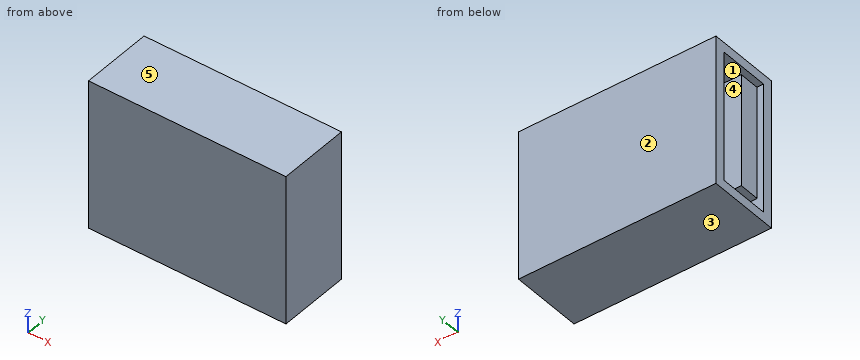
```python
from build123d import *

# Parameters (mm, degrees)
F0_W     = 19.3
F0_H     = 14.6
F1_DEPTH = 7
F2_W     = 5
F2_H     = 12.7
F3_DEPTH = 10
F4_W     = 2
F4_H     = 11
F5_DEPTH = 10


with BuildPart() as f1:
    # F0 (on Front) → F1 (new body)
    with BuildSketch(Plane.XZ):
        with Locations((9.65, 7.3)):
            Rectangle(F0_W, F0_H)
    extrude(amount=F1_DEPTH)

    # F2 (on face) → F3 (cut)
    with BuildSketch(Plane(origin=(0, 0, 0), x_dir=(0, -1, 0), z_dir=(-1, 0, 0))):
        with Locations((3.5, 7.3)):
            Rectangle(F2_W, F2_H)
    extrude(amount=-F3_DEPTH, mode=Mode.SUBTRACT)

    # F4 (on face) → F5 (join)
    with BuildSketch(Plane(origin=(10, 0, 0), x_dir=(0, -1, 0), z_dir=(-1, 0, 0))):
        with Locations((4.2, 7.3)):
            Rectangle(F4_W, F4_H)
    extrude(amount=F5_DEPTH)


solid = f1.part
```
Geometry check sheet. Reference: the model listing, model coordinates, mm. Face numbers are marked on the shaded views. A direction names the side the tool comes from. Coordinates: 2 decimals unless noted, no trailing zeros. Write each loop counter-clockwise with the first axis right and the second up, starting at its lowest first coordinate (ties: lowest second). Pieces come first, ordered by that corner, then holes. Notation, with made-up numbers: M 66.5,23 L 103.5,23 A26 cw 103.5,38 Z; hole C 22.25,80 d1. An arc over 180 degrees is marked long. Use one line per item in the form item = value. Start each with the question number.
1) Section check A-A on x = 6.75. Enter the section's corners in (y, z).
2) Section check C-C on z = 9. Enter the section's corners in (x, y).
3) Release check for a two-part mould opening along Z. For the marked faces 1, 2 and 3 record: pulls with the +Z half, pulls with the -Z half, needs draft (parallel to the pull), parting line crosses it, or undercut.
4) Section check D-D on y = -4.5. Enter the section's corners in (x, z).
5) Thickness scan on probe 1 along Z at (x, y) = (4.75, -4.25); probe 2 along Y at (x, z) = (8.25, 11); probe 3 along Y at (x, z) = (4.25, 1). Record the ranges inside material, lowest first. Write a range as from..to.
6) Set-up check for the marked faces 4 and 5: record each of +Z, -Z, +X, -X, +Y, -Y from which the full face is reachable in a straight line by a thin tool's end or side.
7) Section check B-B on y = -2.75. Enter the section's corners in (x, z).
Responses:
q1.outline = M -7,0 L 0,0 L 0,14.6 L -7,14.6 Z; M -5.2,1.8 L -3.2,1.8 L -3.2,12.8 L -5.2,12.8 Z; hole M -6,0.95 L -1,0.95 L -1,13.65 L -6,13.65 Z
q2.outline = M 0,-7 L 19.3,-7 L 19.3,0 L 0,0 L 0,-1 L 10,-1 L 10,-3.2 L 0,-3.2 L 0,-5.2 L 10,-5.2 L 10,-6 L 0,-6 Z
q3.face_1 = undercut
q3.face_2 = needs draft
q3.face_3 = pulls with the -Z half
q4.outline = M 0,0 L 19.3,0 L 19.3,14.6 L 0,14.6 L 0,13.65 L 10,13.65 L 10,12.8 L 0,12.8 L 0,1.8 L 10,1.8 L 10,0.95 L 0,0.95 Z
q5.probe_1 = 0..0.95, 1.8..12.8, 13.65..14.6
q5.probe_2 = -7..-6, -5.2..-3.2, -1..0
q5.probe_3 = -7..-6, -1..0
q6.face_4 = -X
q6.face_5 = +Z, +X, -X, +Y, -Y
q7.outline = M 0,0 L 19.3,0 L 19.3,14.6 L 0,14.6 L 0,13.65 L 10,13.65 L 10,0.95 L 0,0.95 Z
